Part print with two shaded views. Sizes in mm from the minimum x, y, z corner. Give positions to 0.01 mm unless a question says otherwise; leave off trailing zeros. Write each loop counter-clockwise with the first axis right and the second up, starting at its lowest first coordinate (ties: lowest second). Pieces come first, ordered by that corner, then holes.
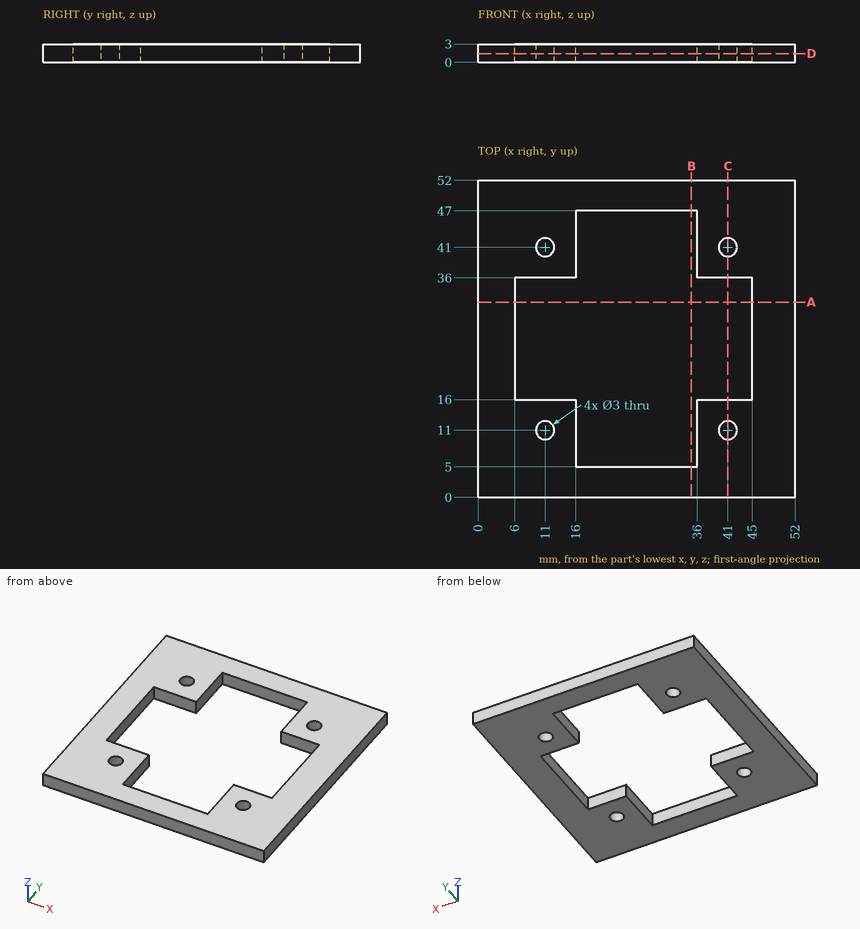
(1) Drop a flat-ended pin along its axis: pin 1 (1.5 mm diameter, centred on y = 10, z = 2, fed in from -X). Give the stop position or say it passes through.
(2) Saw through at C-C, the plane x = 41. List the corners of the cut face in (y, z).
(3) Saw through at D-D, the plane z = 1.4. List the corners of the cut face in (x, y), plus the area to 3 significant figures.
(4) Probe line 1 (Y direction, x = 11, z = 1.7); line 2 (X direction, y = 7.5, z = 2.75). List the from-to ranges inside material, lowest first.
(5) Saw through at A-A, the plane y = 32. List the corners of the cut face in (x, z).
(6) Saw through at B-B, the plane x = 35. List the corners of the cut face in (y, z), plus the area to 3 significant figures.
Computed values:
1. pin 1: stops at x = 0
2. outline: (0, 0) - (9.5, 0) - (9.5, 3) - (0, 3) - close; (12.5, 0) - (16, 0) - (16, 3) - (12.5, 3) - close; (36, 0) - (39.5, 0) - (39.5, 3) - (36, 3) - close; (42.5, 0) - (52, 0) - (52, 3) - (42.5, 3) - close
3. outline: (0, 0) - (52, 0) - (52, 52) - (0, 52) - close; hole (6, 16) - (16, 16) - (16, 5) - (36, 5) - (36, 16) - (45, 16) - (45, 36) - (36, 36) - (36, 47) - (16, 47) - (16, 36) - (6, 36) - close; hole circle Ø3 at (11, 11); hole circle Ø3 at (11, 41); hole circle Ø3 at (41, 11); hole circle Ø3 at (41, 41)
3. area: 1,460 mm2
4. line 1: y = 0 to 9.5, 12.5 to 16, 36 to 39.5, 42.5 to 52
4. line 2: x = 0 to 16, 36 to 52
5. outline: (0, 0) - (6, 0) - (6, 3) - (0, 3) - close; (45, 0) - (52, 0) - (52, 3) - (45, 3) - close
6. outline: (0, 0) - (5, 0) - (5, 3) - (0, 3) - close; (47, 0) - (52, 0) - (52, 3) - (47, 3) - close
6. area: 30.0 mm2
